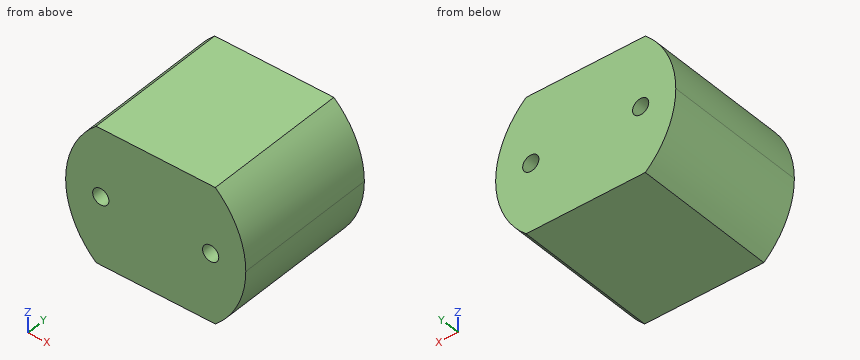
from build123d import *

# Parameters (mm, degrees)
SKETCH1_W                = 25.4
SKETCH1_H                = 25.4
BOSS_EXTRUDE1_DEPTH      = 20.32
SKETCH2_R                = 1.143
CUT_EXTRUDE1_DEPTH       = 28.11977876
FILLET1_R                = 12.7
CUT_EXTRUDE2_START       = -12.7
CUT_EXTRUDE2_OUTLINE_W   = 20
CUT_EXTRUDE2_OUTLINE_H   = 20.32
CUT_EXTRUDE2_DEPTH       = 3.175
CUT_EXTRUDE2_START_2     = 9.525
CUT_EXTRUDE2_2_OUTLINE_W = 20
CUT_EXTRUDE2_2_OUTLINE_H = 20.32
CUT_EXTRUDE2_2_DEPTH     = 3.175


# Read off the part's stored shape, not the designer's step: Cut-Extrude2
with BuildPart() as part:
    # Sketch1 → Boss-Extrude1 (new body)
    with BuildSketch(Plane(origin=(0, 0, 0), x_dir=(1, 0, 0), z_dir=(0, 1, 0))):
        Rectangle(SKETCH1_W, SKETCH1_H)
    extrude(amount=BOSS_EXTRUDE1_DEPTH)

    # Sketch2 → Cut-Extrude1 (cut, through all)
    with BuildSketch(Plane(origin=(0, 20.32, 0), x_dir=(1, 0, 0), z_dir=(0, 1, 0))):
        with Locations(Location((-7.747, 0, 0), (0, 0, 270))):
            Circle(SKETCH2_R)
        with Locations(Location((7.747, 0, 0), (0, 0, 90))):
            Circle(SKETCH2_R)
    extrude(amount=-CUT_EXTRUDE1_DEPTH, mode=Mode.SUBTRACT)

    # Fillet1
    fillet1_edges = [part.edges().sort_by_distance(p)[0] for p in [
        (-12.7, 10.16, -12.7),
        (12.7, 10.16, -12.7),
        (12.7, 10.16, 12.7),
        (-12.7, 10.16, 12.7),
    ]]
    fillet(fillet1_edges, radius=FILLET1_R - 0.0001)  # a hair under: the kernel refuses the full size

    # Cut-Extrude2 outline → Cut-Extrude2 (cut)
    with BuildSketch(Plane.XY.offset(CUT_EXTRUDE2_START)):
        with Locations((0, 10.16)):
            Rectangle(CUT_EXTRUDE2_OUTLINE_W, CUT_EXTRUDE2_OUTLINE_H)
    extrude(amount=CUT_EXTRUDE2_DEPTH, mode=Mode.SUBTRACT)

    # Cut-Extrude2 2 outline → Cut-Extrude2 2 (cut)
    with BuildSketch(Plane.XY.offset(CUT_EXTRUDE2_START_2)):
        with Locations((0, 10.16)):
            Rectangle(CUT_EXTRUDE2_2_OUTLINE_W, CUT_EXTRUDE2_2_OUTLINE_H)
    extrude(amount=CUT_EXTRUDE2_2_DEPTH, mode=Mode.SUBTRACT)


solid = part.part
Work out the finished part from the listing and answer in its coordinate system (mm). Coordinates: 2 decimals unless noted, no trailing zeros. Loops run counter-clockwise (first coordinate to the right, second up) from the corner with the lowest first, then second, coordinate; pieces in that order, holes last. Notation, with made-up numbers: M 75.5,39 L 107.5,39 A19 cw 107.5,71 Z; hole C -15.75,49 d3. An arc over 180 degrees is marked long. Answer in a Markdown table with one row per item. Add a question column.
1. Find section A-A, the plane y = 5.25. State how many separate pieces and enclosed holes the cut face has, then the cut area to 3 significant figures.
2. Find section C-C, the plane z = 5.75. Write down the section's boundary in (x, y), then the cut area to 3 significant figures.
3. Find section B-B, the plane x = 9.5. Write down the section's boundary in (y, z), then the cut area to 3 significant figures.
4. Consider L1, parallel to X at y = 10.75, z = 0; L2, parallel to X at y = 13.5, z = -0.75; L3, parallel to Z at x = 8, y = 18.25 (3 decimals). Determine where each line is inside the solid, lowest interval first.
5. Flat-ended cylindrical pins translate along their axes: P1, Ø2, axis at x = -7.747, z = 0, coming from the +Y side; P2, Ø3, axis at y = 14.5, z = 2, coming from the +X side; P3, Ø4, axis at y = 15, z = -0.5, coming from the -X side; P4, Ø1.5, axis at x = 9.5, y = 6, coming from the +Z side. Find the tip coordinate at first contact, or state that the pin passes through.
Reported:
| question | item | result |
|---|---|---|
| 1 | separate pieces | 1 |
| 1 | enclosed holes | 2 |
| 1 | area | 425 mm^2 |
| 2 | outline | M -11.32,0 L 11.32,0 L 11.32,20.32 L -11.32,20.32 Z |
| 2 | area | 460 mm^2 |
| 3 | outline | M 0,-8.43 L 20.32,-8.43 L 20.32,8.43 L 0,8.43 Z |
| 3 | area | 343 mm^2 |
| 4 | L1 | x = -12.7 to -8.89, -6.6 to 6.6, 8.89 to 12.7 |
| 4 | L2 | x = -12.68 to -8.61, -6.88 to 6.88, 8.61 to 12.68 |
| 4 | L3 | z = -9.525 to -1.115, 1.115 to 9.525 |
| 5 | P1 | passes through |
| 5 | P2 | stops at x = 12.69 |
| 5 | P3 | stops at x = -12.7 |
| 5 | P4 | stops at z = 9.2 |
